Verification items for the finished model (mm, model axes). Round coordinates to 2 decimals unless told otherwise and drop trailing zeros. Order: outer loops, then holes, each group sorted by start corner. A loop starts at its lowest first (then second) coordinate and runs counter-clockwise, first axis right, second up. Notation, with made-up numbers: (-8, 15.25) -> (33, 15.25) arc R22 ccw to (33, 47.25) -> close; hole circle Ø4 at (61, 27.25). An arc over 180 degrees is marked (long way). Return JSON: item names as keys, results as strings. Group by question number.
Item 1: Scan lines: probe 1 along Z at (x, y) = (6.5, 1.3); probe 2 along Z at (x, y) = (-8.25, 1.95); probe 3 along Z at (x, y) = (-6.25, 0.2). Record each from-to range of solid material in increasing order. Write a range as from..to.
Item 2: Sectioned sample at C-C on x = 0. Record the cut outline in (y, z).
Item 3: Sectioned sample at A-A on y = 1.65. Record the cut outline in (x, z), plus the area to 3 significant figures.
Item 4: Sectioned sample at D-D on x = 3.75. Record the cut outline in (y, z), plus the area to 3 significant figures.
Item 5: Depth check by flat-ended pin: pin 1 Ø1.1 at (x, y) = (0.5, 1.5) entering from -Z; pin 2 Ø1.1 at (y, z) = (0.5, 38.5) entering from -X; pin 3 Ø0.5 at (x, y) = (2, 1.5) entering from +Z. Enter the tip coordinate at first touch or a pass-through.
Item 6: Draft check along Z on faces 1 (the flat face through (0, 1, 8)), 2 (the cylindrical face through (0, 0.5, -38)), 3 (the flat face through (1, 2, -15)). Enter one of: pulls with the +Z half, pulls with the -Z half, needs draft (parallel to the pull), parting line crosses it, or undercut.
Item 7: Sectioned sample at B-B on z = -1.5. Record the cut outline in (x, y), plus the area to 3 significant figures.
```python
from build123d import *

# Parameters (mm, degrees)
BOSS_EXTRUDE1_DEPTH = 1
SKETCH2_R           = 2
CUT_EXTRUDE1_DEPTH  = 2
SKETCH4_W           = 18
SKETCH4_H           = 14
SKETCH4_W_2         = 15
SKETCH4_H_2         = 10
SKETCH4_W_3         = 14
BOSS_EXTRUDE2_DEPTH = 1


with BuildPart() as part:
    # Sketch1 → Boss-Extrude1 (new body)
    with BuildSketch(Plane(origin=(0, 0, 0), x_dir=(1, 0, 0), z_dir=(0, 1, 0))):
        with BuildLine():
            Line((11, 40), (-11, 40))
            Line((-11, 40), (-11, -36))
            Line((-11, -36), (-10, -36))
            Line((-10, -36), (-10, -40))
            Line((-10, -40), (-7, -40))
            Line((-7, -40), (-7, -37.2))
            ThreePointArc((-7, -37.2), (-6.794974747, -36.705025253), (-6.3, -36.5))
            Line((-6.3, -36.5), (-6.2, -36.5))
            ThreePointArc((-6.2, -36.5), (-5.705025253, -36.705025253), (-5.5, -37.2))
            Line((-5.5, -37.2), (-5.5, -40))
            Line((-5.5, -40), (10, -40))
            Line((10, -40), (10, -36))
            Line((10, -36), (11, -36))
            Line((11, -36), (11, 40))
        make_face()
    extrude(amount=BOSS_EXTRUDE1_DEPTH)

    # Sketch2 → Cut-Extrude1 (cut, through all)
    with BuildSketch(Plane(origin=(0, 1, 0), x_dir=(1, 0, 0), z_dir=(0, 1, 0))):
        with Locations((0, 40)):
            Circle(SKETCH2_R)
    extrude(amount=-CUT_EXTRUDE1_DEPTH, mode=Mode.SUBTRACT)

    # Sketch4 → Boss-Extrude2 (add)
    with BuildSketch(Plane(origin=(0, 1, 0), x_dir=(1, 0, 0), z_dir=(0, 1, 0))):
        with Locations((0, 29)):
            Rectangle(SKETCH4_W, SKETCH4_H)
        with Locations((1.5, 15)):
            Rectangle(SKETCH4_W_2, SKETCH4_H_2)
        Rectangle(SKETCH4_W_3, SKETCH4_H)
        with Locations((0, -26)):
            Rectangle(SKETCH4_W, SKETCH4_H)
    extrude(amount=BOSS_EXTRUDE2_DEPTH)


solid = part.part
```
Recorded:
{
 "1": {"probe 1": "-36..-22, -20..-10, -7..7, 19..33", "probe 2": "-36..-22, 19..33", "probe 3": "-40..36.5"},
 "2": {"outline": "(0, -38) -> (1, -38) -> (1, -36) -> (2, -36) -> (2, -22) -> (1, -22) -> (1, -20) -> (2, -20) -> (2, -10) -> (1, -10) -> (1, -7) -> (2, -7) -> (2, 7) -> (1, 7) -> (1, 19) -> (2, 19) -> (2, 33) -> (1, 33) -> (1, 40) -> (0, 40) -> close"},
 "3": {"outline": "(-9, -36) -> (9, -36) -> (9, -22) -> (-9, -22) -> close; (-9, 19) -> (9, 19) -> (9, 33) -> (-9, 33) -> close; (-7, -7) -> (7, -7) -> (7, 7) -> (-7, 7) -> close; (-6, -20) -> (9, -20) -> (9, -10) -> (-6, -10) -> close", "area": "850 mm²"},
 "4": {"outline": "(0, -40) -> (1, -40) -> (1, -36) -> (2, -36) -> (2, -22) -> (1, -22) -> (1, -20) -> (2, -20) -> (2, -10) -> (1, -10) -> (1, -7) -> (2, -7) -> (2, 7) -> (1, 7) -> (1, 19) -> (2, 19) -> (2, 33) -> (1, 33) -> (1, 40) -> (0, 40) -> close", "area": "132 mm²"},
 "5": {"pin 1": "z = -38.14", "pin 2": "x = -10", "pin 3": "z = 33"},
 "6": {"face 1": "undercut", "face 2": "pulls with the -Z half", "face 3": "needs draft"},
 "7": {"outline": "(-11, 0) -> (11, 0) -> (11, 1) -> (7, 1) -> (7, 2) -> (-7, 2) -> (-7, 1) -> (-11, 1) -> close", "area": "36.0 mm²"}
}
